Read the model definition and answer for the solid it produces. Units are mm, in the model's axes. A direction names the side the tool comes from. Give positions to 0.01 mm unless a question says otherwise; leave off trailing zeros. Write each loop counter-clockwise with the first axis right and the second up, starting at its lowest first coordinate (ties: lowest second). Pieces come first, ordered by that corner, then holes. Notation, with made-up numbers: M 31,35.25 L 39,35.25 A26 cw 39,54.25 Z; hole C 89,-31 d5. An arc over 180 degrees is marked long. Use a Markdown table: item, result. Add a question column.
Item 1: The mould has two halves that part along X. Classify faces 5 (the flat face through (-23, -4, 3)), 6 (the flat face through (21.5, -20, 5)), 7 (the flat face through (0, -9, 7)), 8 (the flat face through (5.1, -4, 5)): pulls with the +X half, pulls with the -X half, needs draft (parallel to the pull), parting line crosses it, or undercut.
Item 2: For faces 1 (the flat face through (26.5, -20, 4)), 2 (the flat face through (26, -10.8, 6.5)), 3 (the flat face through (-20, -11, 3)), 4 (the flat face through (-2, -5, 3)), determine the directions among +Z, -Z, +X, -X, +Y, -Y from which every point of the face is accessible in a straight line to the end or side of a thin tool.
Item 3: A cutting plane is placed at A-A on x = 0. Determine the outline of the cut face in (y, z).
Item 4: Given P1, Ø3, axis at x = 1, z = 5, coming from the +Y side; P2, Ø2, axis at y = -5, z = 5, coming from the +X side; P3, Ø4, axis at x = -12.5, y = -10, coming from the +Z side, each flat-ended and moving along its own axis, determine where each tip first touches the part or whether it passes through.
Item 5: Consider probe 1 along X at (y, z) = (-26, 7.25); probe 2 along Y at (x, z) = (0, 2.35); probe 3 along Y at (x, z) = (12, 5.25). Determine where each line is inside the solid, lowest interval first. Write a range as [from, to].
Item 6: A cutting plane is placed at C-C on y = -19.75. Determine the outline of the cut face in (x, z), then the cut area to 3 significant figures.
Item 7: A cutting plane is placed at B-B on z = 1.5. Determine the outline of the cut face in (x, y), then the cut area to 3 significant figures.
Item 8: A cutting plane is placed at D-D on x = -14. Determine the outline of the cut face in (y, z).
from build123d import *

# Parameters (mm, degrees)
BOSS_EXTRUDE1_DEPTH  = 7
SKETCH6_W            = 5
SKETCH6_H            = 10
BOSS_EXTRUDE2_DEPTH  = 4
SKETCH3_W            = 5.1
SKETCH3_H            = 7.5
CUT_EXTRUDE1_DEPTH   = 4
M4_CLEARANCE_HOLE1_D = 4.5
CHAMFER2_SIZE        = 4
FILLET2_R            = 3


# Some blends are built 0.0001 mm under size
with BuildPart() as part:
    # Sketch1 → Boss-Extrude1 (new body)
    with BuildSketch(Plane.XY):
        Polygon((0, 0), (0, -10), (-19, -10), (-21.5, -12.5), (-21.5, -27.5), (-26.5, -27.5), (-26.5, -7.5), (-19, 0), align=None)
    boss_extrude1 = extrude(amount=BOSS_EXTRUDE1_DEPTH)

    # Sketch6 → Boss-Extrude2 (add)
    with BuildSketch(Plane.XY.offset(7)):
        with Locations((-24, -22.5)):
            Rectangle(SKETCH6_W, SKETCH6_H)
    boss_extrude2 = extrude(amount=BOSS_EXTRUDE2_DEPTH)

    # Sketch3 → Cut-Extrude1 (cut)
    with BuildSketch(Plane.XY.offset(7)):
        with Locations((-2.55, -3.75)):
            Rectangle(SKETCH3_W, SKETCH3_H)
    cut_extrude1 = extrude(amount=-CUT_EXTRUDE1_DEPTH, mode=Mode.SUBTRACT)

    # Mirror1: Boss-Extrude1, Boss-Extrude2, Cut-Extrude1 across plane
    add(boss_extrude1.mirror(Plane(origin=(0, 0, 7), x_dir=(0, 0, 1), z_dir=(-1, 0, 0))))
    add(boss_extrude2.mirror(Plane(origin=(0, 0, 7), x_dir=(0, 0, 1), z_dir=(-1, 0, 0))))
    add(cut_extrude1.mirror(Plane(origin=(0, 0, 7), x_dir=(0, 0, 1), z_dir=(-1, 0, 0))), mode=Mode.SUBTRACT)

    # M4 Clearance Hole1 (through all)
    with Locations(Plane.XY.offset(3)):
        with Locations((0, -3.5)):
            Hole(M4_CLEARANCE_HOLE1_D / 2)

    # Chamfer2
    chamfer2_edges = [part.edges().sort_by_distance(p)[0] for p in [
        (-24, -17.5, 7),
        (24, -17.5, 7),
    ]]
    chamfer(chamfer2_edges, length=CHAMFER2_SIZE - 0.0001)  # a hair under: the kernel refuses the full size

    # Chamfer4
    # the kernel refuses this chamfer: 1 mm, written as the material it takes off along each edge
    with BuildSketch(Plane(origin=(26.5, -11.68164552, 5.18154552), x_dir=(-0.9996219169112968, 0.019442520806014118, 0.01944252080601436), z_dir=(0, -0.7071067811865476, 0.7071067811865476))) as chamfer4_piece_1_section:
        with BuildLine():
            Line((1.028673195, 0), (-0.056547155, 1.027117794))
            Line((-0.056547155, 1.027117794), (-0.076539593, 1.026567876))
            ThreePointArc((-0.076539593, 1.026567876), (-0.034129227, 0.51339783), (-0.019992438, -0.000549918))
            Line((-0.019992438, -0.000549918), (0.000549918, -0.019992438))
            ThreePointArc((0.000549918, -0.019992438), (0.514497665, -0.00585565), (1.029223113, -0.019992438))
            Line((1.029223113, -0.019992438), (1.028673195, 0))
        make_face()
    chamfer4_piece_1 = extrude(amount=10.800078804, mode=Mode.PRIVATE)
    chamfer4_piece_1 = split(chamfer4_piece_1, bisect_by=Plane(origin=(26.156619069, -15.715277747, 7), z_dir=(0, 0, 1)), keep=Keep.TOP, mode=Mode.PRIVATE)
    add(chamfer4_piece_1, mode=Mode.SUBTRACT)
    with BuildSketch(Plane(origin=(-26.5, -11.68164552, 5.18154552), x_dir=(0.9996219169112968, 0.019442520806013806, 0.019442520806013806), z_dir=(0, -0.7071067811865476, 0.7071067811865476))) as chamfer4_piece_2_section:
        with BuildLine():
            Line((1.028673195, 0), (-0.056547155, -1.027117794))
            Line((-0.056547155, -1.027117794), (-0.076539593, -1.026567876))
            ThreePointArc((-0.076539593, -1.026567876), (-0.034129227, -0.51339783), (-0.019992438, 0.000549918))
            Line((-0.019992438, 0.000549918), (0.000549918, 0.019992438))
            ThreePointArc((0.000549918, 0.019992438), (0.514497665, 0.00585565), (1.029223113, 0.019992438))
            Line((1.029223113, 0.019992438), (1.028673195, 0))
        make_face()
    chamfer4_piece_2 = extrude(amount=10.800078804, mode=Mode.PRIVATE)
    chamfer4_piece_2 = split(chamfer4_piece_2, bisect_by=Plane(origin=(-26.156619069, -15.715277747, 7), z_dir=(0, 0, 1)), keep=Keep.TOP, mode=Mode.PRIVATE)
    add(chamfer4_piece_2, mode=Mode.SUBTRACT)
    with BuildSketch(Plane(origin=(-28.31845448, -9.31845448, 7), x_dir=(0.7068394360706726, -0.7068394360706746, 0.027495876610586528), z_dir=(0.7071067811865485, 0.7071067811865466, 0))) as chamfer4_piece_3:
        with BuildLine():
            Line((1.028673195, 0), (-0.056547155, 1.027117794))
            Line((-0.056547155, 1.027117794), (-0.076539593, 1.026567876))
            ThreePointArc((-0.076539593, 1.026567876), (-0.034129227, 0.51339783), (-0.019992438, -0.000549918))
            Line((-0.019992438, -0.000549918), (0.000549918, -0.019992438))
            ThreePointArc((0.000549918, -0.019992438), (0.514497665, -0.00585565), (1.029223113, -0.019992438))
            Line((1.029223113, -0.019992438), (1.028673195, 0))
        make_face()
    extrude(amount=15.749967694, mode=Mode.SUBTRACT)
    with BuildSketch(Plane(origin=(-26.5, -16.071782988, 7), x_dir=(0.9996219169112968, 0, 0.02749587661058651), z_dir=(0, 1, 0))) as chamfer4_piece_4_section:
        with BuildLine():
            Line((1.028673195, 0), (-0.056547155, 1.027117794))
            Line((-0.056547155, 1.027117794), (-0.076539593, 1.026567876))
            ThreePointArc((-0.076539593, 1.026567876), (-0.034129227, 0.51339783), (-0.019992438, -0.000549918))
            Line((-0.019992438, -0.000549918), (0.000549918, -0.019992438))
            ThreePointArc((0.000549918, -0.019992438), (0.514497665, -0.00585565), (1.029223113, -0.019992438))
            Line((1.029223113, -0.019992438), (1.028673195, 0))
        make_face()
    chamfer4_piece_4 = extrude(amount=11.143465976, mode=Mode.PRIVATE)
    chamfer4_piece_4 = split(chamfer4_piece_4, bisect_by=Plane(origin=(-26.166087376, -11.115587602, 4.615487602), z_dir=(0, 0.7071067811865476, 0.7071067811865476)), keep=Keep.TOP, mode=Mode.PRIVATE)
    add(chamfer4_piece_4, mode=Mode.SUBTRACT)
    with BuildSketch(Plane(origin=(-21.571682988, 0, 7), x_dir=(0, -0.9996219169112968, 0.027495876610586494), z_dir=(1, 0, 0))) as chamfer4_piece_5:
        with BuildLine():
            Line((1.028673195, 0), (-0.056547155, 1.027117794))
            Line((-0.056547155, 1.027117794), (-0.076539593, 1.026567876))
            ThreePointArc((-0.076539593, 1.026567876), (-0.034129227, 0.51339783), (-0.019992438, -0.000549918))
            Line((-0.019992438, -0.000549918), (0.000549918, -0.019992438))
            ThreePointArc((0.000549918, -0.019992438), (0.514497665, -0.00585565), (1.029223113, -0.019992438))
            Line((1.029223113, -0.019992438), (1.028673195, 0))
        make_face()
    extrude(amount=19.043365976, mode=Mode.SUBTRACT)
    with BuildSketch(Plane(origin=(26.5, -16.071782988, 7), x_dir=(-0.9996219169112968, 0, 0.02749587661058651), z_dir=(0, 1, 0))) as chamfer4_piece_6_section:
        with BuildLine():
            Line((1.028673195, 0), (-0.056547155, -1.027117794))
            Line((-0.056547155, -1.027117794), (-0.076539593, -1.026567876))
            ThreePointArc((-0.076539593, -1.026567876), (-0.034129227, -0.51339783), (-0.019992438, 0.000549918))
            Line((-0.019992438, 0.000549918), (0.000549918, 0.019992438))
            ThreePointArc((0.000549918, 0.019992438), (0.514497665, 0.00585565), (1.029223113, 0.019992438))
            Line((1.029223113, 0.019992438), (1.028673195, 0))
        make_face()
    chamfer4_piece_6 = extrude(amount=11.143465976, mode=Mode.PRIVATE)
    chamfer4_piece_6 = split(chamfer4_piece_6, bisect_by=Plane(origin=(26.166087376, -11.115587602, 4.615487602), z_dir=(0, 0.7071067811865476, 0.7071067811865476)), keep=Keep.TOP, mode=Mode.PRIVATE)
    add(chamfer4_piece_6, mode=Mode.SUBTRACT)
    with BuildSketch(Plane(origin=(28.31845448, -9.31845448, 7), x_dir=(-0.7068394360706725, -0.7068394360706747, 0.027495876610586528), z_dir=(-0.7071067811865487, 0.7071067811865464, 0))) as chamfer4_piece_7:
        with BuildLine():
            Line((1.028673195, 0), (-0.056547155, -1.027117794))
            Line((-0.056547155, -1.027117794), (-0.076539593, -1.026567876))
            ThreePointArc((-0.076539593, -1.026567876), (-0.034129227, -0.51339783), (-0.019992438, 0.000549918))
            Line((-0.019992438, 0.000549918), (0.000549918, 0.019992438))
            ThreePointArc((0.000549918, 0.019992438), (0.514497665, 0.00585565), (1.029223113, 0.019992438))
            Line((1.029223113, 0.019992438), (1.028673195, 0))
        make_face()
    extrude(amount=15.749967694, mode=Mode.SUBTRACT)
    with BuildSketch(Plane(origin=(21.571682988, 0, 7), x_dir=(0, -0.9996219169112968, 0.027495876610586494), z_dir=(-1, 0, 0))) as chamfer4_piece_8:
        with BuildLine():
            Line((1.028673195, 0), (-0.056547155, -1.027117794))
            Line((-0.056547155, -1.027117794), (-0.076539593, -1.026567876))
            ThreePointArc((-0.076539593, -1.026567876), (-0.034129227, -0.51339783), (-0.019992438, 0.000549918))
            Line((-0.019992438, 0.000549918), (0.000549918, 0.019992438))
            ThreePointArc((0.000549918, 0.019992438), (0.514497665, 0.00585565), (1.029223113, 0.019992438))
            Line((1.029223113, 0.019992438), (1.028673195, 0))
        make_face()
    extrude(amount=19.043365976, mode=Mode.SUBTRACT)
    with BuildSketch(Plane(origin=(26.5, -16.071782988, 7), x_dir=(-0.9996219169112968, 0, 0.02749587661058651), z_dir=(0, 1, 0))) as chamfer4_piece_9a_section:
        with BuildLine():
            Line((1.028673195, 0), (-0.056547155, -1.027117794))
            Line((-0.056547155, -1.027117794), (-0.076539593, -1.026567876))
            ThreePointArc((-0.076539593, -1.026567876), (-0.034129227, -0.51339783), (-0.019992438, 0.000549918))
            Line((-0.019992438, 0.000549918), (0.000549918, 0.019992438))
            ThreePointArc((0.000549918, 0.019992438), (0.514497665, 0.00585565), (1.029223113, 0.019992438))
            Line((1.029223113, 0.019992438), (1.028673195, 0))
        make_face()
    chamfer4_piece_9a = extrude(amount=11.143465976, mode=Mode.PRIVATE)
    chamfer4_piece_9a = split(chamfer4_piece_9a, bisect_by=Plane(origin=(26.181906875, -13.879260813, 7.379160813), z_dir=(0, -0.7071067811865476, -0.7071067811865476)), keep=Keep.TOP, mode=Mode.PRIVATE)
    with BuildSketch(Plane(origin=(26.5, -11.68164552, 5.18154552), x_dir=(-0.9996219169112968, 0.019442520806014118, 0.01944252080601436), z_dir=(0, -0.7071067811865476, 0.7071067811865476))) as chamfer4_piece_9b_section:
        with BuildLine():
            Line((1.028673195, 0), (-0.056547155, 1.027117794))
            Line((-0.056547155, 1.027117794), (-0.076539593, 1.026567876))
            ThreePointArc((-0.076539593, 1.026567876), (-0.034129227, 0.51339783), (-0.019992438, -0.000549918))
            Line((-0.019992438, -0.000549918), (0.000549918, -0.019992438))
            ThreePointArc((0.000549918, -0.019992438), (0.514497665, -0.00585565), (1.029223113, -0.019992438))
            Line((1.029223113, -0.019992438), (1.028673195, 0))
        make_face()
    chamfer4_piece_9b = extrude(amount=10.800078804, mode=Mode.PRIVATE)
    chamfer4_piece_9b = split(chamfer4_piece_9b, bisect_by=Plane(origin=(26.181906875, -12.963885635, 7), z_dir=(0, 0, -1)), keep=Keep.TOP, mode=Mode.PRIVATE)
    chamfer4_piece_9 = chamfer4_piece_9a & chamfer4_piece_9b
    add(chamfer4_piece_9, mode=Mode.SUBTRACT)
    with BuildSketch(Plane(origin=(-26.5, -16.071782988, 7), x_dir=(0.9996219169112968, 0, 0.02749587661058651), z_dir=(0, 1, 0))) as chamfer4_piece_10a_section:
        with BuildLine():
            Line((1.028673195, 0), (-0.056547155, 1.027117794))
            Line((-0.056547155, 1.027117794), (-0.076539593, 1.026567876))
            ThreePointArc((-0.076539593, 1.026567876), (-0.034129227, 0.51339783), (-0.019992438, -0.000549918))
            Line((-0.019992438, -0.000549918), (0.000549918, -0.019992438))
            ThreePointArc((0.000549918, -0.019992438), (0.514497665, -0.00585565), (1.029223113, -0.019992438))
            Line((1.029223113, -0.019992438), (1.028673195, 0))
        make_face()
    chamfer4_piece_10a = extrude(amount=11.143465976, mode=Mode.PRIVATE)
    chamfer4_piece_10a = split(chamfer4_piece_10a, bisect_by=Plane(origin=(-26.181906875, -13.879260813, 7.379160813), z_dir=(0, -0.7071067811865476, -0.7071067811865476)), keep=Keep.TOP, mode=Mode.PRIVATE)
    with BuildSketch(Plane(origin=(-26.5, -11.68164552, 5.18154552), x_dir=(0.9996219169112968, 0.019442520806013806, 0.019442520806013806), z_dir=(0, -0.7071067811865476, 0.7071067811865476))) as chamfer4_piece_10b_section:
        with BuildLine():
            Line((1.028673195, 0), (-0.056547155, -1.027117794))
            Line((-0.056547155, -1.027117794), (-0.076539593, -1.026567876))
            ThreePointArc((-0.076539593, -1.026567876), (-0.034129227, -0.51339783), (-0.019992438, 0.000549918))
            Line((-0.019992438, 0.000549918), (0.000549918, 0.019992438))
            ThreePointArc((0.000549918, 0.019992438), (0.514497665, 0.00585565), (1.029223113, 0.019992438))
            Line((1.029223113, 0.019992438), (1.028673195, 0))
        make_face()
    chamfer4_piece_10b = extrude(amount=10.800078804, mode=Mode.PRIVATE)
    chamfer4_piece_10b = split(chamfer4_piece_10b, bisect_by=Plane(origin=(-26.181906875, -12.963885635, 7), z_dir=(0, 0, -1)), keep=Keep.TOP, mode=Mode.PRIVATE)
    chamfer4_piece_10 = chamfer4_piece_10a & chamfer4_piece_10b
    add(chamfer4_piece_10, mode=Mode.SUBTRACT)

    # Fillet2
    fillet2_edges = [part.edges().sort_by_distance(p)[0] for p in [
        (-24, -27.5, 11),
        (24, -27.5, 11),
    ]]
    fillet(fillet2_edges, radius=FILLET2_R)


solid = part.part
Filled in:
| question | item | result |
|---|---|---|
| 1 | face 5 | pulls with the -X half |
| 1 | face 6 | undercut |
| 1 | face 7 | needs draft |
| 1 | face 8 | undercut |
| 2 | face 1 | +Z, -Z, +X, +Y, -Y |
| 2 | face 2 | +Z, +X, +Y |
| 2 | face 3 | +Z, -Z, -Y |
| 2 | face 4 | +Z, +Y |
| 3 | outline | M -10,0 L -5.75,0 L -5.75,3 L -7.5,3 L -7.5,7 L -10,7 Z; M -1.25,0 L 0,0 L 0,3 L -1.25,3 Z |
| 4 | P1 | y = -7.5 |
| 4 | P2 | x = 25 |
| 4 | P3 | z = 7 |
| 5 | probe 1 | [-26.5, -21.5], [21.5, 26.5] |
| 5 | probe 2 | [-10, -5.75], [-1.25, 0] |
| 5 | probe 3 | [-10, 0] |
| 6 | outline | M -26.5,0 L -21.5,0 L -21.5,11 L -26.5,11 Z; M 21.5,0 L 26.5,0 L 26.5,11 L 21.5,11 Z |
| 6 | area | 110 mm² |
| 7 | outline | M -26.5,-27.5 L -21.5,-27.5 L -21.5,-12.5 L -19,-10 L 19,-10 L 21.5,-12.5 L 21.5,-27.5 L 26.5,-27.5 L 26.5,-7.5 L 19,0 L -19,0 L -26.5,-7.5 Z; hole C 0,-3.5 d4.5 |
| 7 | area | 639 mm² |
| 8 | outline | M -10,0 L 0,0 L 0,6 L -1,7 L -10,7 Z |
